Work out the finished part from the listing and answer in its coordinate system (mm). A direction names the side the tool comes from. Give positions to 0.01 mm unless a question says otherwise; leave off trailing zeros. Write each loop counter-clockwise with the first axis right and the second up, starting at its lowest first coordinate (ties: lowest second). Pieces come first, ordered by that corner, then holes.
1) Determine the mould class of faces 1 (the face through (-31.476, 15.535, -9.912)), 2 (the face through (-8.06, 29.58, -12.65)), 3 (the face through (39.92, 47.54, 0.49)), 4 (the face through (-32, 35, -32)) for opening direction X: pulls with the +X half, pulls with the -X half, needs draft (parallel to the pull), parting line crosses it, or undercut.
2) Find section A-A (y = 51.5). Determine the outline of the cut face in (x, z), plus the area to 3 significant figures.
3) Given pin 1 Ø1.5 at (y, z) = (48.5, 42.5) entering from -X; pin 2 Ø6 at (x, z) = (32, 29.5) entering from +Y; pin 3 Ø8 at (y, z) = (12, 11.5) entering from +X, each flat-ended and moving along its own axis, determine where each tip first touches the part or whether it passes through.
4) A tool of negligible diameter and unlimited length cuts with its end or side. For faces 5 (the face through (-27.791, 40.07, -38.398)), 6 (the face through (27.791, 40.07, 38.398)), 7 (the face through (-39.92, 47.54, -0.49)), from which of +Z, -Z, +X, -X, +Y, -Y can it reach the whole face along a straight path? Write none if from no direction.
5) Find section B-B (z = -48.5). Determine the outline of the cut face in (x, y), plus the area to 3 significant figures.
6) Straight lines are drawn through the part: probe 1 along Y at (x, z) = (-17, 37); probe 2 along Y at (x, z) = (26.5, -28); probe 3 along Y at (x, z) = (-16, -48). For each, find the intervals that lie inside material, in ascending order.
```python
from build123d import *

# Parameters (mm, degrees)
SKETCH3_R                = 35
BOSS_EXTRUDE1_DEPTH      = 5
BOSS_EXTRUDE3_DEPTH      = 10
FILLET1_R                = 10
SKETCH5_R                = 3.5
CUT_EXTRUDE1_DEPTH       = 15
CIRPATTERN1_COUNT        = 4
FILLET1_OF_CIRPATTERN1_R = 10


with BuildPart() as part:
    # Sketch1 → Revolve1 (revolve)
    with BuildSketch(Plane.XY, mode=Mode.PRIVATE) as revolve1_sk:
        Polygon((15, 60), (15, 0), (30, 0), (31.763269807, -10), (36, -10), (37.763269807, 0), (37.763269807, 5), (60, 5), (60, 13), (33, 13), (33, 18), (35, 18), (35, 60), (33, 60), (33, 55), (30, 55), (30, 60), (25.386751346, 60), (22.5, 55), (19.613248654, 60), align=None)
    revolve(revolve1_sk.sketch.rotate(Axis((0, 25.612491422, 0), (0, -1, 0)), 180), axis=Axis((0, 25.612491422, 0), (0, -1, 0)))  # turned: the seam where the file's is

    # Sketch3 → Boss-Extrude1 (add)
    with BuildSketch(Plane(origin=(0, 50, 0), x_dir=(1, 0, 0), z_dir=(0, 1, 0))):
        with BuildLine():
            ThreePointArc((44.062305213, 35.018621544), (42.072853481, 42.072853481), (35.018621544, 44.062305213))
            ThreePointArc((35.018621544, 44.062305213), (0, 39.917357046), (-35.018621544, 44.062305213))
            ThreePointArc((-35.018621544, 44.062305213), (-42.072853481, 42.072853481), (-44.062305213, 35.018621544))
            ThreePointArc((-44.062305213, 35.018621544), (-39.917357046, 0), (-44.062305213, -35.018621544))
            ThreePointArc((-44.062305213, -35.018621544), (-42.072853481, -42.072853481), (-35.018621544, -44.062305213))
            ThreePointArc((-35.018621544, -44.062305213), (0, -39.917357046), (35.018621544, -44.062305213))
            ThreePointArc((35.018621544, -44.062305213), (42.072853481, -42.072853481), (44.062305213, -35.018621544))
            ThreePointArc((44.062305213, -35.018621544), (39.917357046, 0), (44.062305213, 35.018621544))
        make_face()
        with Locations(Location((0, 0, 0), (0, 0, 180))):  # turned: the seam where the file's is
            Circle(SKETCH3_R, mode=Mode.SUBTRACT)
    extrude(amount=-BOSS_EXTRUDE1_DEPTH)

    # Sketch4 → Boss-Extrude3 (add)
    with BuildSketch(Plane.XZ.offset(-45)):
        with BuildLine():
            Line((29.477150366, 18.870548648), (42.072853481, 31.466251763))
            ThreePointArc((42.072853481, 31.466251763), (42.072853481, 42.072853481), (31.466251763, 42.072853481))
            Line((31.466251763, 42.072853481), (18.870548648, 29.477150366))
            ThreePointArc((18.870548648, 29.477150366), (24.748737342, 24.748737342), (29.477150366, 18.870548648))
        make_face()
    boss_extrude3 = extrude(amount=BOSS_EXTRUDE3_DEPTH)

    # Fillet1
    fillet1_edges = [part.edges().sort_by_distance(p)[0] for p in [
        (18.870548648, 40, 29.477150366),
        (29.477150366, 40, 18.870548648),
    ]]
    fillet(fillet1_edges, radius=FILLET1_R)

    # Sketch5 → Cut-Extrude1 (cut)
    with BuildSketch(Plane(origin=(0, 50, 0), x_dir=(1, 0, 0), z_dir=(0, 1, 0))):
        with Locations(Location((36.769552622, -36.769552622, 0), (0, 0, 180))):  # turned: the seam where the file's is
            Circle(SKETCH5_R)
    cut_extrude1 = extrude(amount=-CUT_EXTRUDE1_DEPTH, mode=Mode.SUBTRACT)

    # CirPattern1: Boss-Extrude3, Cut-Extrude1 ×4 about axis
    cirpattern1_axis = Axis((0, 0, 0), (0, 1, 0))
    add([boss_extrude3.rotate(cirpattern1_axis, i * 360 / CIRPATTERN1_COUNT) for i in range(1, CIRPATTERN1_COUNT)])
    add([cut_extrude1.rotate(cirpattern1_axis, i * 360 / CIRPATTERN1_COUNT) for i in range(1, CIRPATTERN1_COUNT)], mode=Mode.SUBTRACT)

    # Fillet1 of CirPattern1
    fillet1_of_cirpattern1_edges = [part.edges().sort_by_distance(p)[0] for p in [
        (29.477150366, 40, -18.870548648),
        (18.870548648, 40, -29.477150366),
        (-18.870548648, 40, -29.477150366),
        (-29.477150366, 40, -18.870548648),
        (-29.477150366, 40, 18.870548648),
        (-18.870548648, 40, 29.477150366),
    ]]
    fillet(fillet1_of_cirpattern1_edges, radius=FILLET1_OF_CIRPATTERN1_R)


solid = part.part
```
Results:
1. face 1: parting line crosses it
1. face 2: undercut
1. face 3: pulls with the +X half
1. face 4: needs draft
2. outline: circle Ø70 at (0, 0); hole circle Ø30 at (0, 0)
2. area: 3,140 mm2
3. pin 1: stops at x = -42.38
3. pin 2: stops at y = 50
3. pin 3: stops at x = 59.53
4. face 5: -Z
4. face 6: +Z
4. face 7: -X, +Y
5. outline: (-35.32, 5) - (35.32, 5) - (35.32, 13) - (-35.32, 13) - close
5. area: 565 mm2
6. probe 1: y = 5 to 13, 45 to 50
6. probe 2: y = 5 to 13, 35 to 50
6. probe 3: y = 5 to 13
